```python
from build123d import *

# Parameters (mm, degrees)
BOSS_EXTRUDE1_DEPTH = 19
SKETCH3_W           = 4.925645198
SKETCH3_H           = 33.799871634
BOSS_EXTRUDE2_DEPTH = 19
SKETCH4_W           = 4.925645198
SKETCH4_H           = 7.649871634
CUT_EXTRUDE1_DEPTH  = 41.8379487
SKETCH5_W           = 10.925645198
SKETCH5_H           = 26.15
CUT_EXTRUDE3_DEPTH  = 37.834770316
SKETCH6_W           = 24.5
SKETCH6_H           = 6.25
BOSS_EXTRUDE3_DEPTH = 19
SKETCH7_W           = 18
SKETCH7_H           = 64
BOSS_EXTRUDE4_DEPTH = 19
BOSS_EXTRUDE5_DEPTH = 19
SKETCH10_W          = 12.5
SKETCH10_H          = 22.9
CUT_EXTRUDE4_DEPTH  = 16
SKETCH11_W          = 4
SKETCH11_H          = 3
BOSS_EXTRUDE6_DEPTH = 7
SKETCH12_R          = 0.9375
CUT_EXTRUDE5_DEPTH  = 6.5
BOSS_EXTRUDE7_DEPTH = 19
CUT_EXTRUDE6_DEPTH  = 102.016783878
CUT_EXTRUDE7_DEPTH  = 102.016783878
CUT_EXTRUDE8_DEPTH  = 102.016783878
SKETCH20_W          = 9.2
SKETCH20_H          = 10.4
CUT_EXTRUDE10_DEPTH = 102.016783878
SKETCH21_W          = 5
SKETCH21_H          = 22
BOSS_EXTRUDE8_DEPTH = 19
CUT_EXTRUDE11_DEPTH = 102.016783878
CUT_EXTRUDE12_DEPTH = 102.016783878
SKETCH24_W          = 9
SKETCH24_H          = 4
CUT_EXTRUDE13_DEPTH = 10


with BuildPart() as part:
    # Sketch2 → Boss-Extrude1 (new body)
    with BuildSketch(Plane(origin=(0, 0, 0), x_dir=(0, 0, -1), z_dir=(1, 0, 0))):
        Polygon((-4.2, 3.125), (-14.2, 3.125), (-14.2, -3.125), (-4.2, -3.125), (-4.2, -5.2), (-2.4, -5.2), (0, -2.8), (0, 2.8), (-2.4, 5.2), (-4.2, 5.2), align=None)
    boss_extrude1 = extrude(amount=BOSS_EXTRUDE1_DEPTH)

    # Sketch3 → Boss-Extrude2 (add)
    with BuildSketch(Plane.ZY):
        with Locations((16.662822599, 13.774935817)):
            Rectangle(SKETCH3_W, SKETCH3_H)
    extrude(amount=-BOSS_EXTRUDE2_DEPTH)

    # Mirror2: Boss-Extrude1 across plane
    add(boss_extrude1.mirror(Plane.ZX.offset(9.95)))

    # Sketch4 → Cut-Extrude1 (cut, through all)
    with BuildSketch(Plane.ZY):
        with Locations((16.662822599, 26.849935817)):
            Rectangle(SKETCH4_W, SKETCH4_H)
    extrude(amount=-CUT_EXTRUDE1_DEPTH, mode=Mode.SUBTRACT)

    # Sketch5 → Cut-Extrude3 (cut, through all)
    with BuildSketch(Plane(origin=(19, 0, 0), x_dir=(0, 0, -1), z_dir=(1, 0, 0))):
        with Locations((-13.662822599, 9.95)):
            Rectangle(SKETCH5_W, SKETCH5_H)
    extrude(amount=-CUT_EXTRUDE3_DEPTH, mode=Mode.SUBTRACT)


with BuildPart() as cut_extrude3_piece_1:
    # of the separate pieces the step leaves, piece 1, a body of its own (cut_extrude3_pieces)
    add(part.part.solids().sort_by_distance((0, 16.775, 8.2))[0])



with BuildPart() as cut_extrude3_piece_2:
    # of the separate pieces the step leaves, piece 2, a body of its own (cut_extrude3_pieces)
    add(part.part.solids().sort_by_distance((0, 3.125, 4.2))[0])


with BuildPart() as cut_extrude3_piece_1_1:
    add(cut_extrude3_piece_1.part)

    add(cut_extrude3_piece_2.part)  # Boss-Extrude3 merges Cut-Extrude3 piece 2
    # Sketch6 → Boss-Extrude3 (add)
    with BuildSketch(Plane(origin=(19, 0, 0), x_dir=(0, 0, -1), z_dir=(1, 0, 0))):
        Polygon((-25.005276382, 16.775), (-32.7, 16.775), (-8.2, -3.125), (-8.2, 3.125), align=None)
        with Locations((-20.45, 19.9)):
            Rectangle(SKETCH6_W, SKETCH6_H)
    extrude(amount=-BOSS_EXTRUDE3_DEPTH)

    # Sketch7 → Boss-Extrude4 (add)
    with BuildSketch(Plane.ZY):
        with Locations((32.7, 55.025)):
            Rectangle(SKETCH7_W, SKETCH7_H)
    extrude(amount=-BOSS_EXTRUDE4_DEPTH)

    # Sketch9 → Boss-Extrude5 (add)
    with BuildSketch(Plane.ZY):
        Polygon((41.7, 23.025), (32.7, 23.025), (32.7, 16.775), align=None)
    extrude(amount=-BOSS_EXTRUDE5_DEPTH)

    # Sketch10 → Cut-Extrude4 (cut)
    with BuildSketch(Plane.ZY):
        with Locations((32.7, 74.475)):
            Rectangle(SKETCH10_W, SKETCH10_H)
    extrude(amount=-CUT_EXTRUDE4_DEPTH, mode=Mode.SUBTRACT)

    # Sketch11 → Boss-Extrude6 (add)
    with BuildSketch(Plane.ZY):
        with Locations((32.7, 88.525)):
            Rectangle(SKETCH11_W, SKETCH11_H)
    extrude(amount=-BOSS_EXTRUDE6_DEPTH)

    # Sketch12 → Cut-Extrude5 (cut)
    with BuildSketch(Plane.ZY):
        with Locations((32.7, 87.925)):
            Circle(SKETCH12_R)
        with Locations((32.7, 61.025)):
            Circle(SKETCH12_R)
    extrude(amount=-CUT_EXTRUDE5_DEPTH, mode=Mode.SUBTRACT)

    # Sketch13 → Boss-Extrude7 (add)
    with BuildSketch(Plane.ZY):
        Polygon((9.2, 16.775), (9.2, 3.937244898), (25.005276382, 16.775), align=None)
    extrude(amount=-BOSS_EXTRUDE7_DEPTH)

    # Sketch14 → Cut-Extrude6 (cut, through all)
    with BuildSketch(Plane.ZY):
        Polygon((23.7, 59.525), (28.7, 52.275), (28.7, 30.275), (23.7, 23.025), align=None)
        Polygon((36.7, 30.275), (41.7, 23.025), (41.7, 59.525), (36.7, 52.275), align=None)
    extrude(amount=-CUT_EXTRUDE6_DEPTH, mode=Mode.SUBTRACT)

    # Sketch16 → Cut-Extrude7 (cut, through all)
    with BuildSketch(Plane(origin=(19, 0, 0), x_dir=(0, 0, -1), z_dir=(1, 0, 0))):
        Polygon((-8.2, -3.125), (-41.231348669, 23.704544429), (-41.7, 23.025), align=None)
    extrude(amount=-CUT_EXTRUDE7_DEPTH, mode=Mode.SUBTRACT)

    # Sketch17 → Cut-Extrude8 (cut, through all)
    with BuildSketch(Plane.ZY):
        Polygon((36.7, 30.275), (36.7, 20.023979592), (41.231348669, 23.704544429), align=None)
    extrude(amount=-CUT_EXTRUDE8_DEPTH, mode=Mode.SUBTRACT)

    # Sketch20 → Cut-Extrude10 (cut, through all)
    with BuildSketch(Plane.ZY):
        Polygon((36.7, 16.775), (9.2, 16.775), (9.2, 5.2), (9.2, -5.2), (36.7, -5.2), align=None)
        with Locations((4.6, 0)):
            Rectangle(SKETCH20_W, SKETCH20_H)
    extrude(amount=-CUT_EXTRUDE10_DEPTH, mode=Mode.SUBTRACT)

    # Sketch21 → Boss-Extrude8 (add, through all)
    with BuildSketch(Plane.ZY):
        with Locations((8.8, 5.775)):
            Rectangle(SKETCH21_W, SKETCH21_H)
    extrude(amount=-BOSS_EXTRUDE8_DEPTH)

    # Sketch22 → Cut-Extrude11 (cut, through all)
    with BuildSketch(Plane.ZY):
        Polygon((32.7, 16.775), (36.7, 22.575), (36.7, 20.023979592), align=None)
    extrude(amount=-CUT_EXTRUDE11_DEPTH, mode=Mode.SUBTRACT)

    # Sketch23 → Cut-Extrude12 (cut, through all)
    with BuildSketch(Plane.ZY):
        Polygon((23.7, 59.525), (41.7, 59.525), (41.7, -5.225), (6.3, -5.225), (0, 17.1), (0, 22.7), (2.4, 25.1), align=None)
    extrude(amount=-CUT_EXTRUDE12_DEPTH, mode=Mode.SUBTRACT)

    # Sketch24 → Cut-Extrude13 (cut)
    with BuildSketch(Plane.ZY.offset(-16)):
        with Locations((32.7, 65.025)):
            Rectangle(SKETCH24_W, SKETCH24_H)
    extrude(amount=-CUT_EXTRUDE13_DEPTH, mode=Mode.SUBTRACT)


solid = cut_extrude3_piece_1_1.part
```
For this review, take the finished solid that the model builds, in its own axes (mm). A direction names the side the tool comes from. Give positions to 0.01 mm unless a question says otherwise; leave off trailing zeros. Order: outer loops, then holes, each group sorted by start corner. A loop starts at its lowest first (then second) coordinate and runs counter-clockwise, first axis right, second up.
1) Take a section at A-A (z = 32.7). Give the boundary of the cut face in (x, y) (1 decimal), then the cut area to 3 significant figures.
2) Take a section at B-B (y = 66). Give the boundary of the cut face in (x, z).
3) Take a section at C-C (x = 8.5). Give the boundary of the cut face in (y, z) (3 decimals).
4) Take a section at D-D (z = 38). Give the boundary of the cut face in (x, y) (3 decimals).
5) For faces 1 (the face through (3, 89, 34.7)), 2 (the face through (17, 67.025, 33)), 3 (the face through (9, 59.525, 33)), 4 (the face through (9, 63.025, 33)), list the 3-axis set-ups (+Z, -Z, +X, -X, +Y, -Y) from which the entire face can be reached by the end or side of a thin tool; tool diameter is ignored.
6) Wall thickness on line 1 (Y direction, x = 2.5, z = 32.7) (1 decimal); line 2 (Y direction, x = 16.75, z = 31.5) (3 decimals); line 3 (Y direction, x = 5, z = 28.5) (3 decimals): over which ranges is each line inside the solid? List them lowest first.
7) Insertion check: pin 1 (1.5 mm diameter, centred on y = 87.925, z = 32.7, fed in from +X); pin 2 (10 mm diameter, centred on x = 14, z = 31.5, fed in from +Y) (3 decimals); pin 3 (1 mm diameter, centred on y = 73.5, z = 36.5, fed in from -X). Each pin has a flat end and moves straight along its axis. Give the tip position at first contact, or say it passes through.
8) The part is to be moulded in two halves that separate along Z. For faces 5 (the face through (3, 89, 30.7)), 6 (the face through (3.204, 87.566, 33.566)), 7 (the face through (7, 89, 33)), say which applies: released by +Z, released by -Z, zero draft, split by the parting line, or undercut.
Derived:
1. outline: (0, 59.5) - (19, 59.5) - (19, 63) - (0, 63) - (0, 62) - (6.5, 62) - (6.5, 60.1) - (0, 60.1) - close; (0, 85.9) - (16, 85.9) - (16, 67) - (19, 67) - (19, 87) - (7, 87) - (7, 90) - (0, 90) - (0, 88.9) - (6.5, 88.9) - (6.5, 87) - (0, 87) - close
1. area: 141 mm2
2. outline: (0, 23.7) - (19, 23.7) - (19, 28.2) - (16, 28.2) - (16, 26.45) - (0, 26.45) - close; (0, 38.95) - (16, 38.95) - (16, 37.2) - (19, 37.2) - (19, 41.7) - (0, 41.7) - close
3. outline: (59.525, 23.7) - (87.025, 23.7) - (87.025, 41.7) - (59.525, 41.7) - close; hole (63.025, 26.45) - (85.925, 26.45) - (85.925, 38.95) - (63.025, 38.95) - close
4. outline: (0, 59.525) - (19, 59.525) - (19, 87.025) - (0, 87.025) - (0, 85.925) - (16, 85.925) - (16, 63.025) - (0, 63.025) - close
5. face 1: +Z, +X, -X, +Y
5. face 2: +X, -X
5. face 3: +Z, -Z, +X, -X, -Y
5. face 4: -X
6. line 1: y = 59.5 to 60.1, 62 to 63, 85.9 to 87, 88.9 to 90
6. line 2: y = 59.525 to 63.025, 67.025 to 87.025
6. line 3: y = 59.525 to 63.025, 85.925 to 87.025
7. pin 1: stops at x = 7
7. pin 2: stops at y = 87.025
7. pin 3: stops at x = 16
8. face 5: released by -Z
8. face 6: undercut
8. face 7: zero draft
